```python
from build123d import *

# Parameters (mm, degrees)
SKETCH1_R               = 25.4
BOSS_EXTRUDE1_DEPTH     = 38.1
SKETCH2_R               = 50.8
BOSS_EXTRUDE2_DEPTH     = 25.4
SKETCH3_R               = 38.1
BOSS_EXTRUDE3_DEPTH     = 101.6
BOSS_EXTRUDE4_START     = -76.2
BOSS_EXTRUDE4_DEPTH     = 76.2
CUT_EXTRUDE1_REACH      = 316.552
CUT_EXTRUDE1_END_RADIUS = 50.8
SKETCH5_W               = 68.464599232
SKETCH5_H               = 81.28
SKETCH5_R               = 31.75
CUT_EXTRUDE2_REACH      = 310.247
CUT_EXTRUDE2_END_RADIUS = 50.8
SKETCH6_W               = 81.28
SKETCH6_H               = 68.58
SKETCH6_R               = 31.75
SKETCH7_R               = 25.4
CUT_EXTRUDE3_DEPTH      = 76.2
SKETCH8_R               = 25.4
CUT_EXTRUDE4_DEPTH      = 76.2
BOSS_EXTRUDE5_DEPTH     = 25.4
BOSS_EXTRUDE5_TAPER     = 40


with BuildPart() as part:
    # Sketch1 → Boss-Extrude1 (new body)
    with BuildSketch(Plane.XY):
        with Locations(Location((0, 0, 0), (0, 0, 180))):
            Circle(SKETCH1_R)
    extrude(amount=BOSS_EXTRUDE1_DEPTH)

    # Sketch2 → Boss-Extrude2 (add)
    with BuildSketch(Plane.XY.offset(38.1)):
        Circle(SKETCH2_R)
    extrude(amount=BOSS_EXTRUDE2_DEPTH)

    # Sketch3 → Boss-Extrude3 (add)
    with BuildSketch(Plane.XY.offset(63.5)):
        Circle(SKETCH3_R)
    extrude(amount=BOSS_EXTRUDE3_DEPTH)

    # Sketch4 → Boss-Extrude4 (add)
    with BuildSketch(Plane.XY.offset(165.1).offset(BOSS_EXTRUDE4_START)):
        with BuildLine():
            Line((37.998495941, 2.779263607), (116.531903161, -61.680521923))
            Line((116.531903161, -61.680521923), (76.244537205, -110.763901435))
            Line((76.244537205, -110.763901435), (-17.420498723, -33.884158898))
            ThreePointArc((-17.420498723, -33.884158898), (21.021777513, -31.775696219), (37.998495941, 2.779263607))
        make_face()
        with BuildLine():
            Line((25.073469731, 28.686775972), (23.972164439, 130.286775972))
            Line((23.972164439, 130.286775972), (-39.412434793, 130.286775972))
            Line((-39.412434793, 130.286775972), (-38.025917527, 2.374783413))
            ThreePointArc((-38.025917527, 2.374783413), (-14.663618724, 35.165157271), (25.073469731, 28.686775972))
        make_face()
    extrude(amount=BOSS_EXTRUDE4_DEPTH)

    # Cut-Extrude1: up to this cylinder (the profile starts outside it)
    cut_extrude1_end = Plane(origin=(0, 0, 166.577275), z_dir=(0, 0, -1)) * Cylinder(CUT_EXTRUDE1_END_RADIUS, 735.704, mode=Mode.PRIVATE)
    # Sketch5 → Cut-Extrude1 (cut, up to the surface)
    with BuildSketch(Plane(origin=(0, 130.286775972, 0), x_dir=(1, 0, 0), z_dir=(0, 1, 0)), mode=Mode.PRIVATE) as cut_extrude1_sk1:
        with Locations((-7.720135177, -127)):
            Rectangle(SKETCH5_W, SKETCH5_H)
        with Locations((-7.720135177, -127)):
            Circle(SKETCH5_R, mode=Mode.SUBTRACT)
    cut_extrude1_tool1 = extrude(cut_extrude1_sk1.sketch, amount=-CUT_EXTRUDE1_REACH, mode=Mode.PRIVATE) - cut_extrude1_end
    add(cut_extrude1_tool1.solids().sort_by_distance((-7.720135, 130.286776, 166.577275))[0], mode=Mode.SUBTRACT)

    # Cut-Extrude2: up to this cylinder (the profile starts outside it)
    cut_extrude2_end = Plane(origin=(0, 0, 166.576531), z_dir=(0, 0, -1)) * Cylinder(CUT_EXTRUDE2_END_RADIUS, 723.094, mode=Mode.PRIVATE)
    # Sketch6 → Cut-Extrude2 (cut, up to the surface)
    with BuildSketch(Plane(origin=(99.87368094, -81.975763963, 0), x_dir=(0, 0, -1), z_dir=(0.7729666064892688, -0.6344467079688128, 0)), mode=Mode.PRIVATE) as cut_extrude2_sk1:
        with Locations((-127, -5.493701383)):
            Rectangle(SKETCH6_W, SKETCH6_H)
        with Locations(Location((-127, -5.493701383, 0), (0, 0, 90))):
            Circle(SKETCH6_R, mode=Mode.SUBTRACT)
    cut_extrude2_tool1 = extrude(cut_extrude2_sk1.sketch, amount=-CUT_EXTRUDE2_REACH, mode=Mode.PRIVATE) - cut_extrude2_end
    add(cut_extrude2_tool1.solids().sort_by_distance((96.38822, -86.222212, 166.576531))[0], mode=Mode.SUBTRACT)

    # Sketch7 → Cut-Extrude3 (cut)
    with BuildSketch(Plane(origin=(99.87368094, -81.975763963, 0), x_dir=(0, 0, -1), z_dir=(0.7729666064892688, -0.6344467079688128, 0))):
        with Locations(Location((-127, -5.493701383, 0), (0, 0, 90))):
            Circle(SKETCH7_R)
    extrude(amount=-CUT_EXTRUDE3_DEPTH, mode=Mode.SUBTRACT)

    # Sketch8 → Cut-Extrude4 (cut)
    with BuildSketch(Plane(origin=(0, 130.286775972, 0), x_dir=(1, 0, 0), z_dir=(0, 1, 0))):
        with Locations(Location((-7.720135177, -127, 0), (0, 0, 270))):
            Circle(SKETCH8_R)
    extrude(amount=-CUT_EXTRUDE4_DEPTH, mode=Mode.SUBTRACT)

    # Sketch10 → Boss-Extrude5 (add)
    with BuildSketch(Plane.XY.offset(165.1)):
        Polygon((32.144869663, 0), (22.729855319, 22.729855319), (0, 32.144869663), (-22.729855319, 22.729855319), (-32.144869663, 0), (-22.729855319, -22.729855319), (0, -32.144869663), (22.729855319, -22.729855319), align=None)
    extrude(amount=BOSS_EXTRUDE5_DEPTH, taper=BOSS_EXTRUDE5_TAPER)


solid = part.part
```
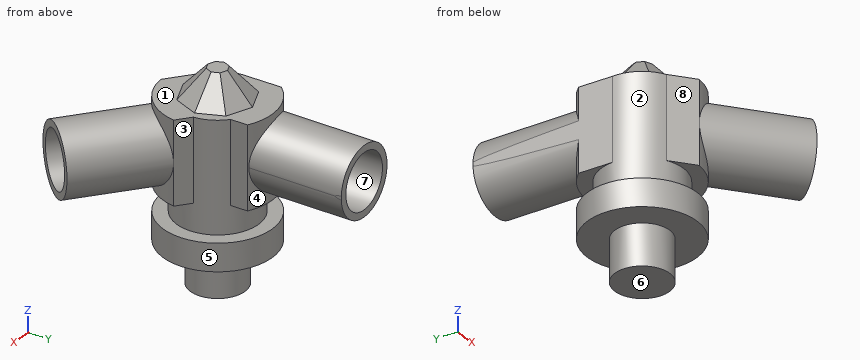
Geometry check sheet. Reference: the model listing, model coordinates, mm. Face numbers are marked on the shaded views. A direction names the side the tool comes from. Coordinates: 2 decimals unless noted, no trailing zeros. Order: outer loops, then holes, each group sorted by start corner. A loop starts at its lowest first (then second) coordinate and runs counter-clockwise, first axis right, second up. Notation, with made-up numbers: M 41,41 L 68,41 A25 cw 68,60 Z; hole C -35,1.25 d3. An arc over 180 degrees is marked long. Answer as a JSON object with one key per item and string values.
Q1. Release check for a two-part mould opening along Z. For the marked faces 6, 7 and 8 record: released by +Z, released by -Z, zero draft, split by the parting line, or undercut.
Results are:
{"face 6": "released by -Z", "face 7": "undercut", "face 8": "zero draft"}
Q2. Scan lines: line 1 (Z direction, x = -7, y = 78.5); line 2 (X direction, y = 104, z = 148); line 3 (Z direction, x = -38, y = -23). Record each from-to range of solid material in increasing order.
Results are:
{"line 1": "z = 95.26 to 101.61, 152.39 to 158.74", "line 2": "x = -31.53 to -22.01, 6.57 to 16.09", "line 3": "z = 38.1 to 63.5"}
Q3. Depth check by flat-ended pin: pin 1 Ø2 at (x, z) = (-8.5, 26) entering from +Y; pin 2 Ø8 at (y, z) = (41.5, 115) entering from -X; pin 3 Ø6 at (y, z) = (-6.5, 47) entering from -X. Enter the tip coordinate at first touch or a pass-through.
Results are:
{"pin 1": "stops at y = 24.27", "pin 2": "stops at x = -38.45", "pin 3": "stops at x = -50.68"}
Q4. Cross-section at A-A on z = 108.5. Record the cut outline in (x, y).
Results are:
{"outline": "M -38.36,33.3 L -38.03,2.37 A38.1 ccw -17.42,-33.88 L 3.08,-50.71 A50.8 ccw 11.07,-49.58 L 80.02,-106.17 L 85.35,-99.68 L 26.45,-51.33 L 48.53,-24.42 L 107.43,-72.77 L 112.76,-66.28 L 48.88,-13.84 A50.8 ccw 50.27,-7.3 L 38,2.78 A38.1 ccw 25.07,28.69 L 24.9,44.28 A50.8 ccw 18.08,47.47 L 18.08,130.29 L 9.68,130.29 L 9.68,54.09 L -25.12,54.09 L -25.12,130.29 L -33.52,130.29 L -33.52,38.17 A50.8 ccw Z"}
Q5. Tool access check on the marked faces 1, 2, 3, 4 and 5. Record the directions out of +Z, -Z, +X, -X, +Y, -Y that give a thin tool (end or side, any length) a straight path to the whole face; none if there is none.
Results are:
{"face 1": "+Z", "face 2": "none", "face 3": "+Z, +X, +Y", "face 4": "+Y", "face 5": "-Z"}
Q6. Cross-section at B-B on y = 98.5. Record the cut outline in (x, z).
Results are:
{"outline": "M -39.07,121.96 A31.75 ccw long -39.07,132.04 Z; hole C -7.72,127 d50.8"}
Q7. Cross-section at C-C on z = 177. Record the cut outline in (x, y), and give its area (3 significant figures).
Results are:
{"outline": "M -21.34,0 L -15.09,-15.09 L 0,-21.34 L 15.09,-15.09 L 21.34,0 L 15.09,15.09 L 0,21.34 L -15.09,15.09 Z", "area": "1,290 mm²"}
